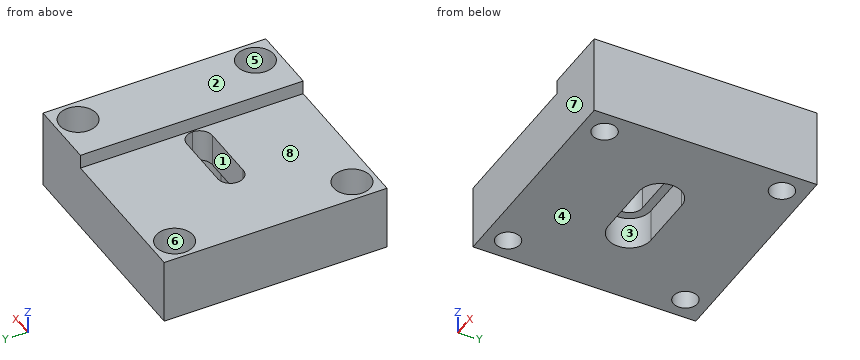
from build123d import *

# Parameters (mm, degrees)
F0_W     = 12.319
F0_H     = 39.878
F0_R     = 3.302
F0_W_2   = 27.559
F1_DEPTH = 11.684
F0_R_2   = 2.159
F2_DEPTH = 5.842
F3_DEPTH = 14.224
F5_DEPTH = 25.4
F6_DEPTH = 5.842


# Not quite as in the source:
# - a feature names something its author has since deleted; it is built from what else it names


with BuildPart() as f1:
    # F0 (on Top) → F1 (new body)
    with BuildSketch(Plane.XY):
        with Locations((13.7795, 0)):
            Rectangle(F0_W, F0_H)
        with Locations((15.875, -15.875)):
            Circle(F0_R, mode=Mode.SUBTRACT)
        with Locations((15.875, 15.875)):
            Circle(F0_R, mode=Mode.SUBTRACT)
        with Locations((-6.1595, 0)):
            Rectangle(F0_W_2, F0_H)
        with Locations((-15.875, -15.875)):
            Circle(F0_R, mode=Mode.SUBTRACT)
        with Locations((-15.875, 15.875)):
            Circle(F0_R, mode=Mode.SUBTRACT)
    extrude(amount=F1_DEPTH)

    # F0 (on Top) → F2 (join)
    with BuildSketch(Plane.XY):
        with Locations((-15.875, 15.875)):
            Circle(F0_R)
        with Locations((-15.875, 15.875)):
            Circle(F0_R_2, mode=Mode.SUBTRACT)
        with Locations((15.875, 15.875)):
            Circle(F0_R)
        with Locations((15.875, 15.875)):
            Circle(F0_R_2, mode=Mode.SUBTRACT)
        with Locations((15.875, -15.875)):
            Circle(F0_R)
        with Locations((15.875, -15.875)):
            Circle(F0_R_2, mode=Mode.SUBTRACT)
        with Locations((-15.875, -15.875)):
            Circle(F0_R)
        with Locations((-15.875, -15.875)):
            Circle(F0_R_2, mode=Mode.SUBTRACT)
    extrude(amount=F2_DEPTH)

    # F0 (on Top) → F3 (join)
    with BuildSketch(Plane.XY):
        with Locations((13.7795, 0)):
            Rectangle(F0_W, F0_H)
        with Locations((15.875, -15.875)):
            Circle(F0_R, mode=Mode.SUBTRACT)
        with Locations((15.875, 15.875)):
            Circle(F0_R, mode=Mode.SUBTRACT)
    extrude(amount=F3_DEPTH)

    # F4 (on face) → F5 (cut)
    with BuildSketch(Plane(origin=(0, 0, 0), x_dir=(1, 0, 0), z_dir=(0, 0, -1))):
        with BuildLine():
            ThreePointArc((-2.794, 0), (-3.4635538982, 1.6164461018), (-5.08, 2.286))
            ThreePointArc((-5.08, 2.286), (-7.366, 0), (-5.08, -2.286))
            ThreePointArc((-5.08, -2.286), (-3.4635538982, -1.6164461018), (-2.794, 0))
        make_face()
        with BuildLine():
            ThreePointArc((7.366, 0), (6.6964461018, 1.6164461018), (5.08, 2.286))
            ThreePointArc((5.08, 2.286), (2.794, 0), (5.08, -2.286))
            ThreePointArc((5.08, -2.286), (6.6964461018, -1.6164461018), (7.366, 0))
        make_face()
        with BuildLine():
            ThreePointArc((-1.27, 0), (-1.4655166344, 1.2048277885), (-2.032, 2.286))
            Line((-2.032, 2.286), (-5.08, 2.286))
            ThreePointArc((-5.08, 2.286), (-3.4635538982, 1.6164461018), (-2.794, 0))
            ThreePointArc((-2.794, 0), (-3.4635538982, -1.6164461018), (-5.08, -2.286))
            Line((-5.08, -2.286), (-2.032, -2.286))
            ThreePointArc((-2.032, -2.286), (-1.4655166344, -1.2048277885), (-1.27, 0))
        make_face()
        with BuildLine():
            ThreePointArc((2.032, -2.286), (1.27, 0), (2.032, 2.286))
            Line((2.032, 2.286), (-2.032, 2.286))
            ThreePointArc((-2.032, 2.286), (-1.4655166344, 1.2048277885), (-1.27, 0))
            ThreePointArc((-1.27, 0), (-1.4655166344, -1.2048277885), (-2.032, -2.286))
            Line((-2.032, -2.286), (2.032, -2.286))
        make_face()
        with BuildLine():
            Line((5.08, 2.286), (2.032, 2.286))
            ThreePointArc((2.032, 2.286), (1.27, 0), (2.032, -2.286))
            Line((2.032, -2.286), (5.08, -2.286))
            ThreePointArc((5.08, -2.286), (2.794, 0), (5.08, 2.286))
        make_face()
    extrude(amount=-F5_DEPTH, mode=Mode.SUBTRACT)

    # F4 (on face) → F6 (cut)
    with BuildSketch(Plane(origin=(0, 0, 0), x_dir=(1, 0, 0), z_dir=(0, 0, -1))):
        with BuildLine():
            ThreePointArc((-1.27, 0), (-1.4655166344, 1.2048277885), (-2.032, 2.286))
            Line((-2.032, 2.286), (-5.08, 2.286))
            ThreePointArc((-5.08, 2.286), (-3.4635538982, 1.6164461018), (-2.794, 0))
            ThreePointArc((-2.794, 0), (-3.4635538982, -1.6164461018), (-5.08, -2.286))
            Line((-5.08, -2.286), (-2.032, -2.286))
            ThreePointArc((-2.032, -2.286), (-1.4655166344, -1.2048277885), (-1.27, 0))
        make_face()
        with BuildLine():
            ThreePointArc((-2.032, 2.286), (-3.3761162011, 3.4077675977), (-5.08, 3.81))
            ThreePointArc((-5.08, 3.81), (-8.89, 0), (-5.08, -3.81))
            ThreePointArc((-5.08, -3.81), (-3.3761162011, -3.4077675977), (-2.032, -2.286))
            Line((-2.032, -2.286), (-5.08, -2.286))
            ThreePointArc((-5.08, -2.286), (-7.366, 0), (-5.08, 2.286))
            Line((-5.08, 2.286), (-2.032, 2.286))
        make_face()
        with BuildLine():
            ThreePointArc((2.032, 2.286), (3.3761162011, 3.4077675977), (5.08, 3.81))
            Line((5.08, 3.81), (-5.08, 3.81))
            ThreePointArc((-5.08, 3.81), (-3.3761162011, 3.4077675977), (-2.032, 2.286))
            Line((-2.032, 2.286), (2.032, 2.286))
        make_face()
        with BuildLine():
            ThreePointArc((2.032, -2.286), (1.27, 0), (2.032, 2.286))
            Line((2.032, 2.286), (-2.032, 2.286))
            ThreePointArc((-2.032, 2.286), (-1.4655166344, 1.2048277885), (-1.27, 0))
            ThreePointArc((-1.27, 0), (-1.4655166344, -1.2048277885), (-2.032, -2.286))
            Line((-2.032, -2.286), (2.032, -2.286))
        make_face()
        with BuildLine():
            Line((5.08, 2.286), (2.032, 2.286))
            ThreePointArc((2.032, 2.286), (1.27, 0), (2.032, -2.286))
            Line((2.032, -2.286), (5.08, -2.286))
            ThreePointArc((5.08, -2.286), (2.794, 0), (5.08, 2.286))
        make_face()
        with BuildLine():
            ThreePointArc((5.08, -3.81), (7.7740768363, -2.6940768363), (8.89, 0))
            ThreePointArc((8.89, 0), (7.7740768363, 2.6940768363), (5.08, 3.81))
            ThreePointArc((5.08, 3.81), (3.3761162011, 3.4077675977), (2.032, 2.286))
            Line((2.032, 2.286), (5.08, 2.286))
            ThreePointArc((5.08, 2.286), (6.6964461018, 1.6164461018), (7.366, 0))
            ThreePointArc((7.366, 0), (6.6964461018, -1.6164461018), (5.08, -2.286))
            Line((5.08, -2.286), (2.032, -2.286))
            ThreePointArc((2.032, -2.286), (3.3761162011, -3.4077675977), (5.08, -3.81))
        make_face()
        with BuildLine():
            Line((-5.08, -3.81), (5.08, -3.81))
            ThreePointArc((5.08, -3.81), (3.3761162011, -3.4077675977), (2.032, -2.286))
            Line((2.032, -2.286), (-2.032, -2.286))
            ThreePointArc((-2.032, -2.286), (-3.3761162011, -3.4077675977), (-5.08, -3.81))
        make_face()
    extrude(amount=-F6_DEPTH, mode=Mode.SUBTRACT)


solid = f1.part
CAD build for the part. Positions are in the model's coordinates, mm. Face numbers are marked on the shaded views. A direction names the side the tool comes from. Give positions to 0.01 mm unless a question says otherwise; leave off trailing zeros. Loops run counter-clockwise (first coordinate to the right, second up) from the corner with the lowest first, then second, coordinate; pieces in that order, holes last. Notation, with made-up numbers: M 6.25,55.25 L 39.25,55.25 A21 ccw 39.25,69.25 Z; hole C -34,54.5 d8. An arc over 180 degrees is marked long. Answer in a Markdown table with one row per item. Add a question column.
Item 1: Band-saw the part on A-A on x = 3. Give the cut face in (y, z), then the cut area to 3 significant figures.
Item 2: Band-saw the part on D-D on y = 5.5. Give the cut face in (x, z).
Item 3: Band-saw the part on C-C on z = 9.75. Give the cut face in (x, y) (3 decimals).
Item 4: Drop flat-ended pins along their axis: P1, Ø3, axis at y = -5.5, z = 13.5, coming from the -X side; P2, Ø2, axis at x = 4.5, y = 1.5, coming from the +Z side; P3, Ø6, axis at x = -4, y = 0.5, coming from the -Z side. Give the stop position or say it passes through.
Item 5: Mould opens along Y. For the marked faces 6, 7 and 8 say: +Y half, -Y half, draft (parallel to the pull), parting line (faces both ways), or undercut.
Item 6: Band-saw the part on B-B on y = 17.5. Give the cut face in (x, z).
Item 7: Tool access for the marked faces 1, 2, 3, 4 and 5: list every direction of +Z, -Z, +X, -X, +Y, -Y with a clear straight run to the whole face (end or side of a thin tool).
Item 8: Probe probe 1 along Y at (x, z) = (-16, 6.25); probe 2 along Y at (x, z) = (16.5, 4.75); probe 3 along Z at (x, y) = (3.5, 3.5). List the from-to ranges inside material, lowest first.
Reply:
| question | item | result |
|---|---|---|
| 1 | outline | M -19.94,0 L -3.81,0 L -3.81,5.84 L -2.29,5.84 L -2.29,11.68 L -19.94,11.68 Z; M 2.29,5.84 L 3.81,5.84 L 3.81,0 L 19.94,0 L 19.94,11.68 L 2.29,11.68 Z |
| 1 | area | 395 mm^2 |
| 2 | outline | M -19.94,0 L 19.94,0 L 19.94,14.22 L 7.62,14.22 L 7.62,11.68 L -19.94,11.68 Z |
| 3 | outline | M -19.939,-19.939 L 19.939,-19.939 L 19.939,19.939 L -19.939,19.939 Z; hole C -15.875,-15.875 d6.604; hole C -15.875,15.875 d6.604; hole M -5.08,-2.286 L 5.08,-2.286 A2.286 ccw 5.08,2.286 L -5.08,2.286 A2.286 ccw Z; hole C 15.875,-15.875 d6.604; hole C 15.875,15.875 d6.604 |
| 4 | P1 | stops at x = 7.62 |
| 4 | P2 | stops at z = 11.68 |
| 4 | P3 | stops at z = 5.84 |
| 5 | face 6 | undercut |
| 5 | face 7 | -Y half |
| 5 | face 8 | draft |
| 6 | outline | M -19.94,0 L -17.3,0 L -17.3,5.84 L -18.75,5.84 L -18.75,11.68 L -19.94,11.68 Z; M -14.45,0 L 14.45,0 L 14.45,5.84 L 13,5.84 L 13,14.22 L 7.62,14.22 L 7.62,11.68 L -13,11.68 L -13,5.84 L -14.45,5.84 Z; M 17.3,0 L 19.94,0 L 19.94,14.22 L 18.75,14.22 L 18.75,5.84 L 17.3,5.84 Z |
| 7 | face 1 | +Z, -Z |
| 7 | face 2 | +Z, +X, -X, +Y, -Y |
| 7 | face 3 | -Z |
| 7 | face 4 | -Z, +X, -X, +Y, -Y |
| 7 | face 5 | +Z |
| 8 | probe 1 | y = -19.94 to -19.17, -12.58 to 12.58, 19.17 to 19.94 |
| 8 | probe 2 | y = -19.94 to -17.94, -13.81 to 13.81, 17.94 to 19.94 |
| 8 | probe 3 | z = 5.84 to 11.68 |
